Could you check a few things on this drawing? It's one solid part, dimensions in mm from its lowest x, y, z. A direction names the side the tool comes from. Round coordinates to 2 decimals unless told otherwise and drop trailing zeros. Order: outer loops, then holes, each group sorted by start corner. A loop starts at its lowest first (then second) coordinate and runs counter-clockwise, first axis right, second up. Notation, with made-up numbers: (-23, 57) - (25, 57) arc R34 cw to (25, 92) - close; hole circle Ø4 at (75, 49.25). An arc over 180 degrees is marked (long way). Use one line per item in the form item = value.
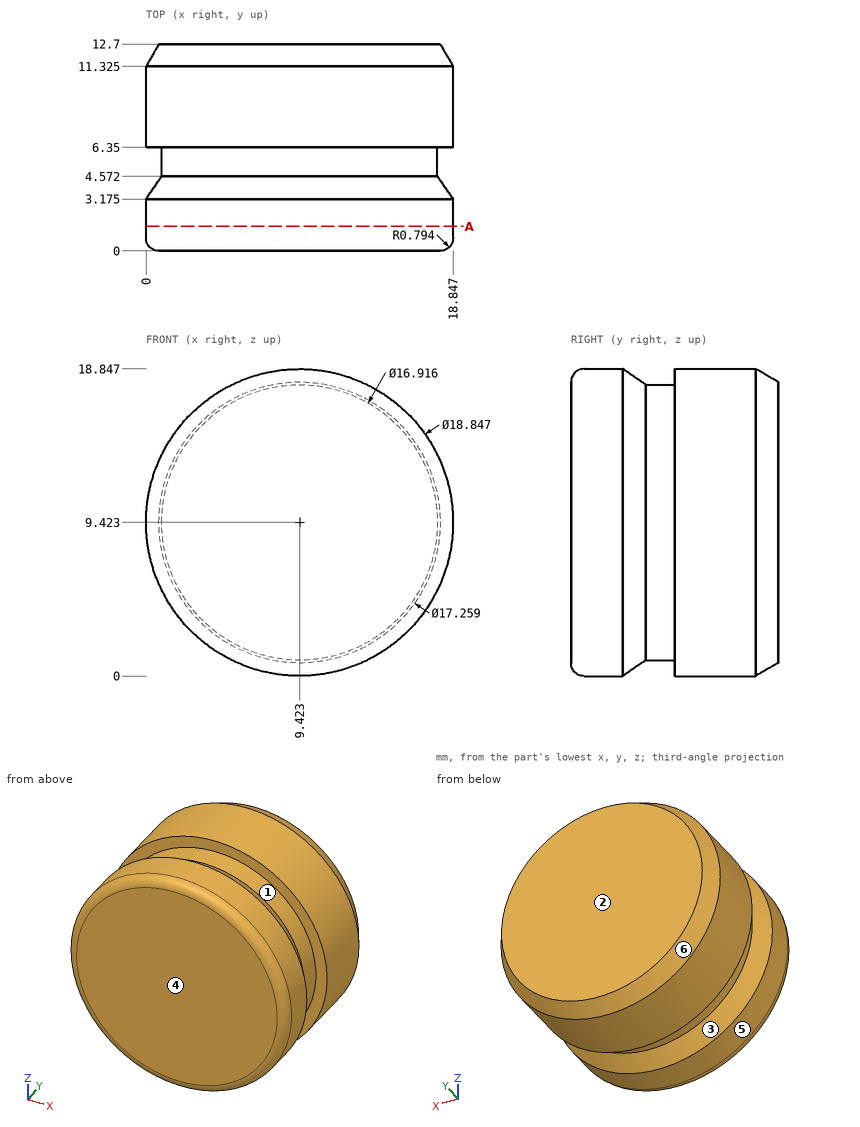
Item 1: If we mould it in two halves opening along Y, with no side actions, what happens to the marked faces 3, 4, 5 and 6? For each: released by +Y, released by -Y, zero draft, split by the parting line, or undercut.
Found:
face_3 = undercut
face_4 = released by -Y
face_5 = zero draft
face_6 = released by +Y
Item 2: For the marked faces 1 and 2, which set-ups out of +Z, -Z, +X, -X, +Y, -Y let a thin tool reach every point of the face, with its end or its side?
Found:
face_1 = none
face_2 = +Z, -Z, +X, -X, +Y
Item 3: Imagine slicing it at A-A on y = 1.5. Please give me the cut outline in (x, z), plus the area to 3 significant figures.
Found:
outline = circle Ø18.85 at (9.42, 9.42)
area = 279 mm2
Item 4: Will these pins go through, and if not, where does the flat tip stop? P1, Ø1.5, axis at x = 16, y = 6.5, coming from the +Z side; P2, Ø1, axis at x = 14.5, y = 8, coming from the -Z side (1 decimal).
Found:
P1 = 16.83
P2 = 1.2
Item 5: I need wall thicknesses on L1, parallel to Z at x = 13, y = 11.75 (1 decimal); L2, parallel to X at y = 3, z = 9.5; L3, parallel to Y at x = 14.5, z = 16.25. Which ranges of each line are inside material? Lowest first, please.
Found:
L1 = 1 to 17.9
L2 = 0 to 18.85
L3 = 0 to 4.5, 6.35 to 12.7
